For this review, take the finished solid that the model builds, in its own axes (mm). A direction names the side the tool comes from. Coordinates: 2 decimals unless noted, no trailing zeros. Write each loop counter-clockwise with the first axis right and the second up, starting at its lowest first coordinate (ties: lowest second). Pieces come first, ordered by that corner, then holes.
```python
from build123d import *

# Parameters (mm, degrees)
SALIENTE_EXTRUIR1_DEPTH = 149
CHAFL_N1_SIZE           = 5
CROQUIS2_R              = 30
CORTAR_EXTRUIR1_DEPTH   = 20


with BuildPart() as part:
    # Croquis1 → Saliente-Extruir1 (new body)
    with BuildSketch(Plane.XY):
        with BuildLine():
            Line((0, 59), (70, 59))
            Line((70, 59), (70, -59))
            Line((70, -59), (0, -59))
            ThreePointArc((0, -59), (-59, 0), (0, 59))
        make_face()
    extrude(amount=SALIENTE_EXTRUIR1_DEPTH)

    # Chaflán1
    chafl_n1_edges = [part.edges().sort_by_distance(p)[0] for p in [
        (70, 0, 149),
        (35, 59, 149),
        (-59, 0, 149),
        (35, -59, 149),
    ]]
    chamfer(chafl_n1_edges, length=CHAFL_N1_SIZE)

    # Croquis2 → Cortar-Extruir1 (cut)
    with BuildSketch(Plane.XY.offset(149)):
        Circle(CROQUIS2_R)
    extrude(amount=-CORTAR_EXTRUIR1_DEPTH, mode=Mode.SUBTRACT)


solid = part.part
```
Q1. Draft analysis for pull direction X (two halves, no side actions). For faces 3 (the flat face through (0, 0, 129)), 4 (the flat face through (35, 56, 147)), 5 (the flat face through (67, 1, 147)), state which applies: +X half, -X half, draft (parallel to the pull), parting line (faces both ways), or undercut.
Ans:
face 3: undercut
face 4: draft
face 5: +X half
Q2. For probe 1 along Y at (x, z) = (0, 135.75); probe 2 along Z at (x, y) = (-3, -19); probe 3 along X at (y, z) = (-1.5, 112.5), list the stretches that pass through material, from the lowest coordinate up.
Ans:
probe 1: y = -59 to -30, 30 to 59
probe 2: z = 0 to 129
probe 3: x = -58.98 to 70
Q3. Tool access review of faces 1 (the cylindrical face through (-29.97, 1.32, 139.14)), 2 (the conical face through (-54.23, -1.193, 148.757)): name each direction out of +Z, -Z, +X, -X, +Y, -Y from which nothing blocks a thin tool from reaching the whole face with its end or side.
Ans:
face 1: +Z
face 2: +Z, -X
Q4. Add section B-B (x = 14). State the section outline as (y, z) points.
Ans:
outline: (-59, 0) - (59, 0) - (59, 144) - (54, 149) - (26.53, 149) - (26.53, 129) - (-26.53, 129) - (-26.53, 149) - (-54, 149) - (-59, 144) - close
Q5. Add section C-C (z = 39). State the section outline as (x, y) points.
Ans:
outline: (0, -59) - (70, -59) - (70, 59) - (0, 59) arc R59 ccw to start
Q6. Add section A-A (y = 0). State the section outline as (x, z) points.
Ans:
outline: (-59, 0) - (70, 0) - (70, 144) - (65, 149) - (30, 149) - (30, 129) - (-30, 129) - (-30, 149) - (-54, 149) - (-59, 144) - close
